Drawing for the job (mm, zero at the part's lowest x, y, z). A direction names the side the tool comes from. Coordinates: 2 decimals unless noted, no trailing zeros. Write each loop counter-clockwise with the first axis right and the second up, starting at its lowest first coordinate (ties: lowest second). Pieces come first, ordered by that corner, then holes. Notation, with made-up numbers: (-17, 86.25) -> (-3, 86.25) arc R18 cw to (-3, 100.25) -> close; hole circle Ø2 at (22, 36). An arc over 180 degrees is marked (long way). Answer as CSV lines item,"result". Start each with the question number.
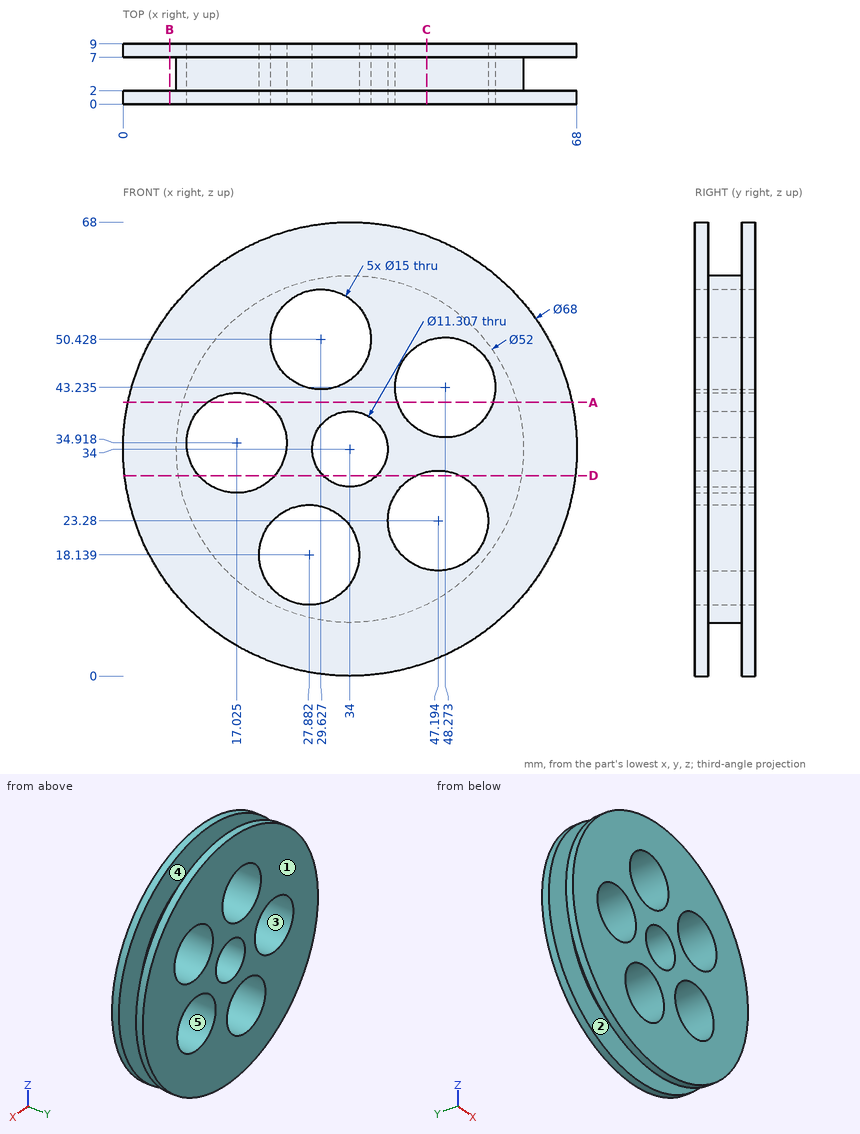
1. Cut at A-A (z = 41). Give the cut face in (x, y), then the cut area to 3 significant figures.
2. Cut at B-B (x = 7). Give the cut face in (y, z), then the cut area to 3 significant figures.
3. Mould opens along Y. For the marked faces 1, 2 and 3 say: pulls with the +Y half, pulls with the -Y half, needs draft (parallel to the pull), parting line crosses it, or undercut.
4. Flat gauge pins, fed straight in: P1, Ø4, axis at x = 61, y = 7.5, coming from the -Z side (1 decimal); P2, Ø4, axis at x = 26, y = 1.5, coming from the +Z side; P3, Ø5, axis at y = 6, z = 59.5, coming from the +X side (1 decimal). Where does each tip first touch, or does it go through?
5. Cut at D-D (z = 30). Give the cut face in (x, y) (1 decimal), then the cut area to 3 significant figures.
6. Tool access for the marked faces 4 and 5: list every direction of +Z, -Z, +X, -X, +Y, -Y with a clear straight run to the whole face (end or side of a thin tool).
7. Wall check: line 1 (Y direction, x = 41.5, z = 65); line 2 (Z direction, x = 36, y = 4.25) (1 decimal); line 3 (X direction, y = 3.25, z = 34) (1 decimal). Give the ranges that are in metal, low to high.
8. Cut at C-C (x = 45.5). Give the cut face in (y, z) (1 decimal).
Geometry check:
1,outline,"(0.73, 0) -> (12.64, 0) -> (12.64, 9) -> (0.73, 9) -> (0.73, 7) -> (8.96, 7) -> (8.96, 2) -> (0.73, 2) -> close; (21.41, 0) -> (41.11, 0) -> (41.11, 9) -> (21.41, 9) -> close; (55.43, 0) -> (67.27, 0) -> (67.27, 2) -> (59.04, 2) -> (59.04, 7) -> (67.27, 7) -> (67.27, 9) -> (55.43, 9) -> close"
1,area,"309 mm²"
2,outline,"(0, 13.34) -> (2, 13.34) -> (2, 54.66) -> (0, 54.66) -> close; (7, 13.34) -> (9, 13.34) -> (9, 54.66) -> (7, 54.66) -> close"
2,area,"165 mm²"
3,face 1,"pulls with the +Y half"
3,face 2,"undercut"
3,face 3,"needs draft"
4,P1,"z = 11"
4,P2,"z = 67.47"
4,P3,"x = 58.8"
5,outline,"(0.2, 0) -> (11.4, 0) -> (11.4, 9) -> (0.2, 9) -> (0.2, 7) -> (8.3, 7) -> (8.3, 2) -> (0.2, 2) -> close; (22.7, 0) -> (30, 0) -> (30, 9) -> (22.7, 9) -> close; (38, 0) -> (43.9, 0) -> (43.9, 9) -> (38, 9) -> close; (50.5, 0) -> (67.8, 0) -> (67.8, 2) -> (59.7, 2) -> (59.7, 7) -> (67.8, 7) -> (67.8, 9) -> (50.5, 9) -> close"
5,area,"293 mm²"
6,face 4,"none"
6,face 5,"+Y, -Y"
7,line 1,"0 to 2, 7 to 9"
7,line 2,"8.1 to 28.7, 39.3 to 46.5, 54.4 to 59.9"
7,line 3,"8 to 9.6, 24.5 to 28.3, 39.7 to 60"
8,outline,"(0, 2) -> (2, 2) -> (2, 10.7) -> (7, 10.7) -> (7, 2) -> (9, 2) -> (9, 16) -> (0, 16) -> close; (0, 30.6) -> (9, 30.6) -> (9, 36.3) -> (0, 36.3) -> close; (0, 50.2) -> (9, 50.2) -> (9, 66) -> (7, 66) -> (7, 57.3) -> (2, 57.3) -> (2, 66) -> (0, 66) -> close"
